Here's how the part is built. I have some questions about the finished solid (model axes, mm). Face numbers are marked on the shaded views. A direction names the side the tool comes from. Coordinates: 2 decimals unless noted, no trailing zeros. Write each loop counter-clockwise with the first axis right and the second up, starting at its lowest first coordinate (ties: lowest second). Pieces come first, ordered by that corner, then holes. Notation, with made-up numbers: (37, -10) - (79, -10) arc R25 ccw to (79, 15) - close; hole circle Ø11 at (83.25, 57). An arc over 180 degrees is marked (long way). Answer in a Markdown table with one row per item. Add a question column.
Item 1: Imagine slicing it at C-C (y = 8.25). Please give me the cut outline in (x, z), plus the area to 3 significant figures.
Item 2: Imagine slicing it at B-B (z = 30). Please give me the cut outline in (x, y).
Item 3: Imagine slicing it at D-D (z = 13.5). Please give me the cut outline in (x, y).
Item 4: Imagine slicing it at A-A (x = 15). Please give me the cut outline in (y, z), plus the area to 3 significant figures.
Item 5: If I drill on probe 1 along Y at (x, z) = (9.25, 13); probe 2 along X at (y, z) = (2.25, 9.5); probe 3 along X at (y, z) = (10, 5), over which ranges is the centre line in solid material (lowest first)? Write a range as from..to.
Item 6: I'm going to push flat-ended pins straight in: pin 1 (4.5 mm diameter, centred on x = 4.5, y = 8.5, fed in from +Z); pin 2 (1 mm diameter, centred on x = 15, y = 16, fed in from -Z); pin 3 (1 mm diameter, centred on x = 15.5, y = 1, fed in from -Z). Where does each tip first touch, or does it pass through?
Item 7: We'd pull the mould along X, two halves only. Please class the marked faces 1, 2, 3 and 4: +X half, -X half, draft (parallel to the pull), parting line (faces both ways), or undercut.
Item 8: Which directions (+Z, -Z, +X, -X, +Y, -Y) give clear straight access to the entire face, cutting with the end or side of a thin tool? Please do the marked faces 5 and 6.
from build123d import *

# Parameters (mm, degrees)
F0_W      = 29
F0_H      = 16.5
F1_DEPTH  = 38.5
F2_T      = -2
F3_DEPTH  = 2.25
F4_SIZE   = 2
F5_SIZE   = 2
F6_SIZE   = 0.99999
F8_DEPTH  = 16.501
F10_DEPTH = 2
F11_R     = 2
F12_DEPTH = 2.001
F13_W     = 7.54
F13_H     = 7.25
F13_R     = 1.1
F14_DEPTH = 4.25


# Not quite as in the source:
# - a fillet or chamfer is up to 0.001 mm smaller than in the source, because OpenCascade refuses the exact size


with BuildPart() as f1:
    # F0 (on Top) → F1 (new body)
    with BuildSketch(Plane.XY):
        with Locations((14.5, 8.25)):
            Rectangle(F0_W, F0_H)
    extrude(amount=F1_DEPTH)

    # F2
    f2_openings = [f1.faces().sort_by_distance(p)[0] for p in [
        (14.5, 8.25, 38.5),
    ]]
    offset(amount=F2_T, openings=f2_openings)

    # F3 (add): a face of the model
    f3_faces = [f1.faces().sort_by_distance(p)[0] for p in [
        (14.5, 8.25, 2),
    ]]
    extrude(f3_faces, amount=F3_DEPTH)

    # F4
    f4_edges = [f1.edges().sort_by_distance(p)[0] for p in [
        (0, 0, 19.25),
        (0, 16.5, 19.25),
        (29, 16.5, 19.25),
        (29, 0, 19.25),
    ]]
    chamfer(f4_edges, length=F4_SIZE)

    # F5 (call 1 of 4: OpenCascade refuses the feature's edges together)
    f5_edges = [f1.edges().sort_by_distance(p)[0] for p in [
        (14.5, 16.5, 0),
    ]]
    chamfer(f5_edges, length=F5_SIZE)

    # F5#2 (call 2 of 4)
    f5_2_edges = [f1.edges().sort_by_distance(p)[0] for p in [
        (29, 8.25, 0),
    ]]
    chamfer(f5_2_edges, length=F5_SIZE)

    # F5#3 (call 3 of 4)
    f5_3_edges = [f1.edges().sort_by_distance(p)[0] for p in [
        (14.5, 0, 0),
    ]]
    chamfer(f5_3_edges, length=F5_SIZE)

    # F5#4 (call 4 of 4)
    f5_4_edges = [f1.edges().sort_by_distance(p)[0] for p in [
        (0, 8.25, 0),
    ]]
    chamfer(f5_4_edges, length=F5_SIZE)

    # F6 (size 1 in the source; OpenCascade refuses exactly that, so slightly less here)
    f6_edges = [f1.edges().sort_by_distance(p)[0] for p in [
        (14.5, 16.5, 38.5),
        (0, 8.25, 38.5),
        (14.5, 0, 38.5),
        (29, 8.25, 38.5),
    ]]
    chamfer(f6_edges, length=F6_SIZE)

    # F7 (on face) → F8 (cut, through all)
    with BuildSketch(Plane.XZ):
        Polygon((6.464, 8.664), (6.464, 4.94), (23.536, 4.94), (23.536, 8.664), (17.364, 12.834), (12.635, 12.834), align=None)
    extrude(amount=-F8_DEPTH, mode=Mode.SUBTRACT)

    # F9 (on face) → F10 (cut, through all)
    with BuildSketch(Plane.YZ.offset(29)):
        with BuildLine():
            Line((2, 28.5), (14.5, 28.5))
            ThreePointArc((14.5, 28.5), (8.25, 34.75), (2, 28.5))
        make_face()
        with BuildLine():
            ThreePointArc((11.4572188031, 23.1356503144), (13.6863414867, 25.4163834155), (14.5, 28.5))
            Line((14.5, 28.5), (2, 28.5))
            ThreePointArc((2, 28.5), (2.7914047728, 25.4559503707), (4.9651962066, 23.1828048711))
            ThreePointArc((4.9651962066, 23.1828048711), (8.2336565888, 26.2499142718), (11.4572188031, 23.1356503144))
        make_face()
        with BuildLine():
            ThreePointArc((2, 28.5), (8.25, 34.75), (14.5, 28.5))
            Line((14.5, 28.5), (14.5, 38.5))
            Line((14.5, 38.5), (2, 38.5))
            Line((2, 38.5), (2, 28.5))
        make_face()
        with BuildLine():
            ThreePointArc((11.4600509613, 23), (11.4593428446, 23.0678399383), (11.4572188031, 23.1356503144))
            ThreePointArc((11.4572188031, 23.1356503144), (8.2046045626, 22.2501648618), (4.9651962066, 23.1828048711))
            ThreePointArc((4.9651962066, 23.1828048711), (8.1186123283, 19.751286566), (11.4600509613, 23))
        make_face()
        with BuildLine():
            ThreePointArc((4.9651962066, 23.1828048711), (8.2046045626, 22.2501648618), (11.4572188031, 23.1356503144))
            ThreePointArc((11.4572188031, 23.1356503144), (8.2336565888, 26.2499142718), (4.9651962066, 23.1828048711))
        make_face()
    extrude(amount=-F10_DEPTH, mode=Mode.SUBTRACT)

    # F11 (on face) → F12 (cut, through all)
    with BuildSketch(Plane.YZ.offset(2)):
        with Locations((8.2100509613, 23)):
            Circle(F11_R)
    extrude(amount=-F12_DEPTH, mode=Mode.SUBTRACT)

    # F13 (on face) → F14 (join)
    with BuildSketch(Plane.YZ.offset(2)):
        with Locations((8.25, 7.875)):
            Rectangle(F13_W, F13_H)
        with Locations((8.25, 9)):
            Circle(F13_R, mode=Mode.SUBTRACT)
    extrude(amount=F14_DEPTH)


solid = f1.part
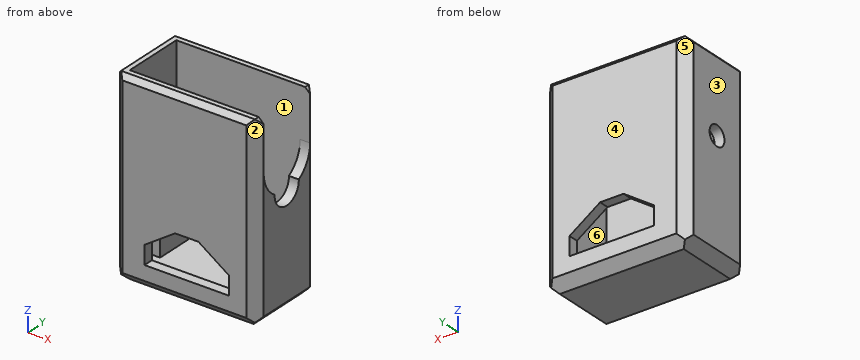
Here are the results:
| question | item | result |
|---|---|---|
| 1 | outline | (0, 2) - (2, 0) - (27, 0) - (29, 2) - (29, 19.75) - (27, 19.75) - (27, 4.25) - (6.25, 4.25) - (6.25, 7.9) - (2, 7.9) - (2, 10.1) - (6.25, 10.1) - (6.25, 11.5) - (2, 11.5) - (2, 21) - (0, 21) - close; (0, 25) - (2, 25) - (2, 38.5) - (1, 38.5) - (0, 37.5) - close |
| 1 | area | 232 mm2 |
| 2 | outline | (0, 2) - (2, 0) - (27, 0) - (29, 2) - (2, 2) - (2, 14.5) - (29, 14.5) - (27, 16.5) - (2, 16.5) - (0, 14.5) - close |
| 3 | outline | (0, 2) - (2, 0) - (27, 0) - (29, 2) - (29, 14.5) - (27, 16.5) - (2, 16.5) - (0, 14.5) - close; hole (2, 2) - (27, 2) - (27, 14.5) - (2, 14.5) - close |
| 4 | outline | (0, 2) - (2, 0) - (14.5, 0) - (16.5, 2) - (16.5, 4.94) - (14.5, 4.94) - (14.5, 4.25) - (2, 4.25) - (2, 4.94) - (0, 4.94) - close; (0, 12.83) - (2, 12.83) - (2, 38.5) - (1, 38.5) - (0, 37.5) - close; (14.5, 12.83) - (16.5, 12.83) - (16.5, 37.5) - (15.5, 38.5) - (14.5, 38.5) - close |
| 4 | area | 171 mm2 |
| 5 | probe 1 | y = 0..2, 14.5..16.5 |
| 5 | probe 2 | x = 0..2, 27..29 |
| 5 | probe 3 | x = 0..6.25, 27..29 |
| 6 | pin 1 | stops at z = 11.5 |
| 6 | pin 2 | stops at z = 1 |
| 6 | pin 3 | stops at z = 0.5 |
| 7 | face 1 | undercut |
| 7 | face 2 | +X half |
| 7 | face 3 | -X half |
| 7 | face 4 | draft |
| 8 | face 5 | +Z, -Z, -X, +Y |
| 8 | face 6 | +Z |
